Build history of the part. All positions in model axes, mm. A direction names the side the tool comes from. Coordinates: 2 decimals unless noted, no trailing zeros. Loops run counter-clockwise (first coordinate to the right, second up) from the corner with the lowest first, then second, coordinate; pieces in that order, holes last.
(1) Slice it at A-A (z = 0). Give the cut face in (x, y) (3 decimals), and give its area (3 significant figures).
(2) Flat gauge pins, fed straight in: P1, Ø3.5, axis at x = 40.6, z = -53.13, coming from the +Y side; P2, Ø3, axis at x = -147, y = 1.5, coming from the +Z side; P3, Ø1.9, axis at x = -95, y = 2, coming from the +Z side; P4, Ø1.9, axis at y = 3.5, z = -19, coming from the -X side. Where does each tip first touch, or does it go through?
(3) Two-plate mould, pull along Z, no slides. Class faces 1 (the face through (-4, 3, -63.5)), 2 (the face through (-44.139, 3.219, -1.514)), 3 (the face through (-46, 0, 13)), 4 (the face through (-65.77, 3.13, -41.89)): pulls with the +Z half, pulls with the -Z half, needs draft (parallel to the pull), parting line crosses it, or undercut.
(4) Tool access for faces 5 (the face through (45.33, 3.22, -61.33)), 6 (the face through (-63.5, 3, -24)): list every direction of +Z, -Z, +X, -X, +Y, -Y with a clear straight run to the whole face (end or side of a thin tool).
(5) Wall check: L1, parallel to X at y = 2.5, z = 1 (3 decimals); L2, parallel to X at y = 2, z = 0 (3 decimals); L3, parallel to Z at x = -113, y = 4.5. Give the ranges that are in metal, low to high.
(6) Slice it at B-B (x = -162.5). Give the cut face in (y, z), and give its area (3 significant figures).
(7) Slice it at C-C (y = 5). Give the number of separate pieces and of enclosed holes in the cut face, and give its area (3 significant figures).
from build123d import *

# Parameters (mm, degrees)
SKETCH1_W           = 95.25
SKETCH1_H           = 127
BOSS_EXTRUDE1_DEPTH = 6.35
BOSS_EXTRUDE3_DEPTH = 6.35
SKETCH5_R           = 4.826
SKETCH5_R_2         = 5.039999953
SKETCH5_R_3         = 1.5
CUT_EXTRUDE1_DEPTH  = 7.35
CUT_EXTRUDE2_DEPTH  = 7.35
FILLET9_R           = 5
FILLET10_R          = 7.62
SKETCH7_R           = 2.2812375
CUT_EXTRUDE3_DEPTH  = 7.35
SKETCH8_R           = 1.830008083
CUT_EXTRUDE4_DEPTH  = 7.35


with BuildPart() as part:
    # Sketch1 → Boss-Extrude1 (new body)
    with BuildSketch(Plane(origin=(0, 0, 0), x_dir=(1, 0, 0), z_dir=(0, 1, 0))):
        Rectangle(SKETCH1_W, SKETCH1_H)
    extrude(amount=BOSS_EXTRUDE1_DEPTH)

    # Sketch4 → Boss-Extrude3 (add)
    with BuildSketch(Plane(origin=(0, 6.35, 0), x_dir=(1, 0, 0), z_dir=(0, 1, 0))):
        with BuildLine():
            Line((-47.625, 63.5), (-171.916018217, 24.219268021))
            ThreePointArc((-171.916018217, 24.219268021), (-189.6618, 0), (-171.916018217, -24.219268021))
            Line((-171.916018217, -24.219268021), (-47.625, -63.5))
            Line((-47.625, -63.5), (-47.625, 63.5))
        make_face()
    extrude(amount=-BOSS_EXTRUDE3_DEPTH)

    # Sketch5 → Cut-Extrude1 (cut, through all)
    with BuildSketch(Plane(origin=(0, 6.35, 0), x_dir=(1, 0, 0), z_dir=(0, 1, 0))):
        with Locations((-164.2618, 0)):
            Circle(SKETCH5_R)
        with Locations((-48.9458, 0)):
            Circle(SKETCH5_R_2)
        with Locations((-40.106965235, 8.838834765)):
            Circle(SKETCH5_R_3)
        with Locations((-57.784634765, -8.838834765)):
            Circle(SKETCH5_R_3)
        with Locations((-55.663314421, 6.717514421)):
            Circle(SKETCH5_R_3)
        with Locations((-42.228285579, -6.717514421)):
            Circle(SKETCH5_R_3)
    extrude(amount=-CUT_EXTRUDE1_DEPTH, mode=Mode.SUBTRACT)

    # Sketch6 → Cut-Extrude2 (cut, through all)
    with BuildSketch(Plane(origin=(0, 6.35, 0), x_dir=(1, 0, 0), z_dir=(0, 1, 0))):
        Polygon((-63.5, 45.163743355), (-157.9118, 6.35), (-63.5, 6.35), align=None)
        Polygon((-63.5, -6.35), (-63.5, -45.163743355), (-157.9118, -6.35), align=None)
    extrude(amount=-CUT_EXTRUDE2_DEPTH, mode=Mode.SUBTRACT)

    # Fillet9
    fillet9_edges = [part.edges().sort_by_distance(p)[0] for p in [
        (-63.5, 3.175, -45.163743355),
        (-63.5, 3.175, -6.35),
        (-157.9118, 3.175, -6.35),
        (-157.9118, 3.175, 6.35),
        (-63.5, 3.175, 6.35),
        (-63.5, 3.175, 45.163743355),
    ]]
    fillet(fillet9_edges, radius=FILLET9_R)

    # Fillet10
    fillet10_edges = [part.edges().sort_by_distance(p)[0] for p in [
        (47.625, 3.175, 63.5),
        (47.625, 3.175, -63.5),
    ]]
    fillet(fillet10_edges, radius=FILLET10_R)

    # Sketch7 → Cut-Extrude3 (cut, through all)
    with BuildSketch(Plane(origin=(0, 6.35, 0), x_dir=(1, 0, 0), z_dir=(0, 1, 0))):
        with Locations((-43.777254611, -53.125383493)):
            Circle(SKETCH7_R)
        with Locations((-43.777254611, 53.125383493)):
            Circle(SKETCH7_R)
        with Locations((40.602254611, 53.125383493)):
            Circle(SKETCH7_R)
        with Locations((40.602254611, -53.125383493)):
            Circle(SKETCH7_R)
    extrude(amount=-CUT_EXTRUDE3_DEPTH, mode=Mode.SUBTRACT)

    # Sketch8 → Cut-Extrude4 (cut, through all)
    with BuildSketch(Plane(origin=(0, 6.35, 0), x_dir=(1, 0, 0), z_dir=(0, 1, 0))):
        with Locations((-6.328465047, -19.828924843)):
            Circle(SKETCH8_R)
        with Locations((-6.328338046, 21.171490961)):
            Circle(SKETCH8_R)
    extrude(amount=-CUT_EXTRUDE4_DEPTH, mode=Mode.SUBTRACT)


solid = part.part
Response values:
1. outline: (-189.662, 0) - (-169.088, 0) - (-169.088, 6.35) - (-189.662, 6.35) - close; (-159.436, 0) - (-53.986, 0) - (-53.986, 6.35) - (-159.436, 6.35) - close; (-43.906, 0) - (47.625, 0) - (47.625, 6.35) - (-43.906, 6.35) - close
1. area: 1,380 mm2
2. P1: passes through
2. P2: stops at z = 32.57
2. P3: stops at z = 48.83
2. P4: stops at x = -182.13
3. face 1: pulls with the -Z half
3. face 2: undercut
3. face 3: needs draft
3. face 4: undercut
4. face 5: -Z, +X, +Y, -Y
4. face 6: +Y, -Y
5. L1: x = -189.642 to -168.983, -159.541 to -53.886, -44.006 to 47.625
5. L2: x = -189.662 to -169.088, -159.436 to -53.986, -43.906 to 47.625
5. L3: z = -42.84 to -24.81, -6.35 to 6.35, 24.81 to 42.84
6. outline: (0, -27.2) - (6.35, -27.2) - (6.35, -4.49) - (0, -4.49) - close; (0, 4.49) - (6.35, 4.49) - (6.35, 27.2) - (0, 27.2) - close
6. area: 288 mm2
7. separate pieces: 1
7. enclosed holes: 14
7. area: 19,900 mm2
